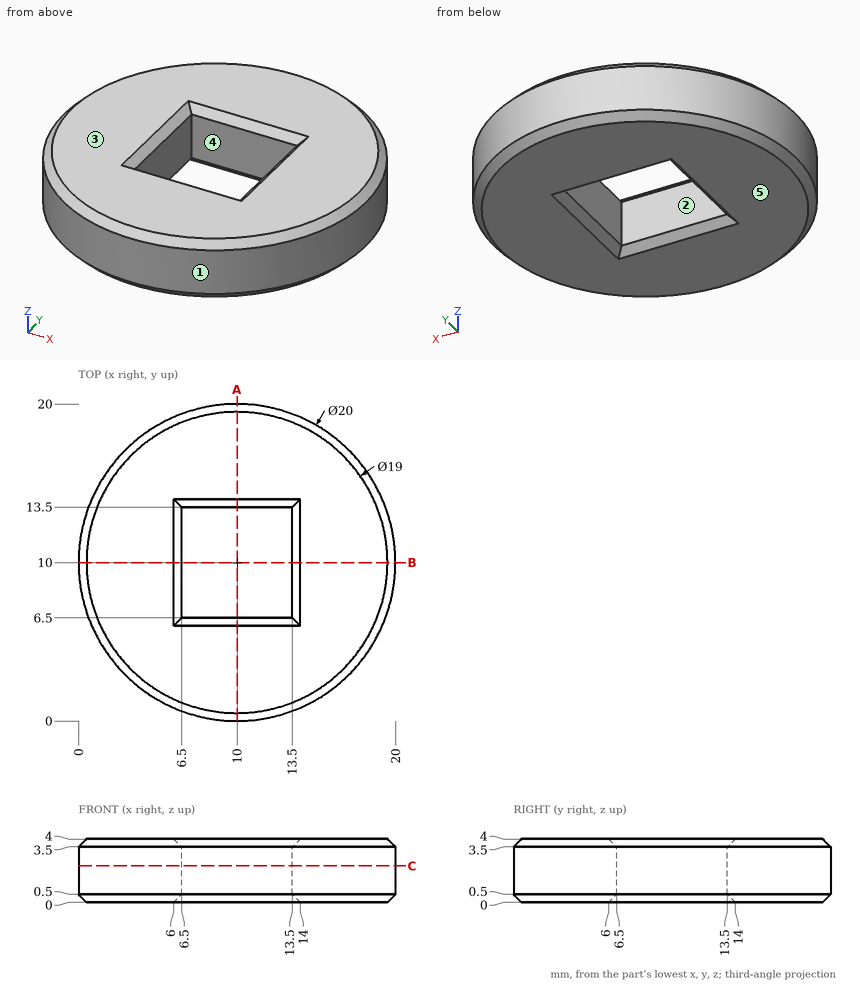
Print and shaded views of the part. All mm, measured from the part's lowest x, y and z. A direction names the side the tool comes from. Coordinates: 2 decimals unless noted, no trailing zeros. Loops run counter-clockwise (first coordinate to the right, second up) from the corner with the lowest first, then second, coordinate; pieces in that order, holes last. Notation, with made-up numbers: M 3,-20.75 L 36,-20.75 A13 ccw 36,-1.75 Z; hole C -27.75,-40 d7. An arc over 180 degrees is marked long. Use a Markdown table: item, result. Add a question column.
Q1. Which spindle directions (+Z, -Z, +X, -X, +Y, -Y) get a long thin tool onto all of the face, cutting with end or side? Do the marked faces 4 and 5. Say none if no direction does.
Q2. Pin check, flat tips, straight feed: P1, Ø1, axis at y = 8, z = 0.5, coming from the +X side; P2, Ø1.5, axis at y = 11.5, z = 1.5, coming from the +X side; P3, Ø1.5, axis at x = 15, z = 2.5, coming from the -Y side. Stop position of each tip, or through.
Q3. Probe L1, parallel to Y at x = 7.25, z = 2.05; L2, parallel to Y at x = 11.75, z = 2.75; L3, parallel to X at y = 5.25, z = 1.6. List the from-to ranges inside material, lowest first.
Q4. Cut at C-C (z = 2.3). Write the cut outline in (x, y).
Q5. Mould opens along X. For the marked faces 1, 2 and 3 say: +X half, -X half, draft (parallel to the pull), parting line (faces both ways), or undercut.
Q6. Cut at A-A (x = 10). Write the cut outline in (y, z), and give its area (3 significant figures).
Worked out:
| question | item | result |
|---|---|---|
| 1 | face 4 | +Z, -Z |
| 1 | face 5 | -Z, +X, -X, +Y, -Y |
| 2 | P1 | stops at x = 19.89 |
| 2 | P2 | stops at x = 19.97 |
| 2 | P3 | stops at y = 0.95 |
| 3 | L1 | y = 0.39 to 6.5, 13.5 to 19.61 |
| 3 | L2 | y = 0.15 to 6.5, 13.5 to 19.85 |
| 3 | L3 | x = 1.2 to 18.8 |
| 4 | outline | C 10,10 d20; hole M 6.5,6.5 L 13.5,6.5 L 13.5,13.5 L 6.5,13.5 Z |
| 5 | face 1 | parting line |
| 5 | face 2 | undercut |
| 5 | face 3 | draft |
| 6 | outline | M 0,0.5 L 0.5,0 L 6,0 L 6.5,0.5 L 6.5,3.5 L 6,4 L 0.5,4 L 0,3.5 Z; M 13.5,0.5 L 14,0 L 19.5,0 L 20,0.5 L 20,3.5 L 19.5,4 L 14,4 L 13.5,3.5 Z |
| 6 | area | 51.0 mm2 |
